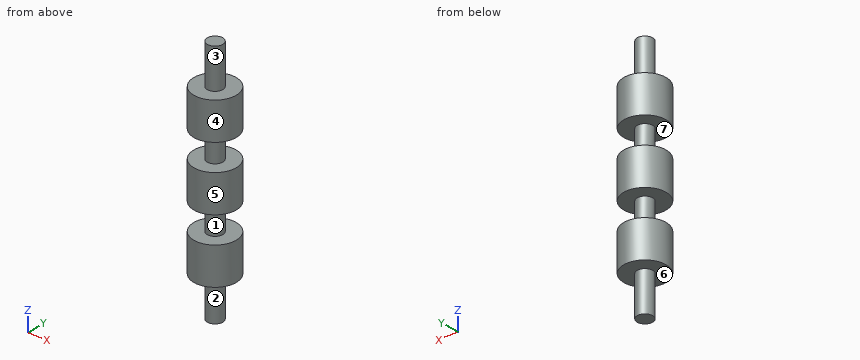
```python
from build123d import *

# Parameters (mm, degrees)
CROQUIS1_R              = 2.95
SALIENTE_EXTRUIR1_DEPTH = 15
CROQUIS2_R              = 8
SALIENTE_EXTRUIR2_DEPTH = 14
SALIENTE_EXTRUIR3_START = 10
CROQUIS3_R              = 2.95
SALIENTE_EXTRUIR3_DEPTH = 10
CROQUIS4_R              = 8
SALIENTE_EXTRUIR4_DEPTH = 14
SALIENTE_EXTRUIR5_START = 10
CROQUIS5_R              = 2.95
SALIENTE_EXTRUIR5_DEPTH = 10
CROQUIS6_R              = 8
SALIENTE_EXTRUIR6_DEPTH = 14
SALIENTE_EXTRUIR7_START = 15
CROQUIS7_R              = 2.95
SALIENTE_EXTRUIR7_DEPTH = 15


with BuildPart() as part:
    # Croquis1 → Saliente-Extruir1 (new body)
    with BuildSketch(Plane.XY):
        Circle(CROQUIS1_R)
    extrude(amount=SALIENTE_EXTRUIR1_DEPTH)

    # Croquis2 → Saliente-Extruir2 (add)
    with BuildSketch(Plane(origin=(0, 0, 0), x_dir=(-1, 0, 0), z_dir=(0, 0, -1))):
        Circle(CROQUIS2_R)
    extrude(amount=SALIENTE_EXTRUIR2_DEPTH)

    # Croquis3 → Saliente-Extruir3 (add)
    with BuildSketch(Plane(origin=(0, 0, -14), x_dir=(-1, 0, 0), z_dir=(0, 0, -1)).offset(SALIENTE_EXTRUIR3_START)):
        with Locations(Location((0, 0, 0), (0, 0, 180))):
            Circle(CROQUIS3_R)
    extrude(amount=-SALIENTE_EXTRUIR3_DEPTH)

    # Croquis4 → Saliente-Extruir4 (add)
    with BuildSketch(Plane(origin=(0, 0, -24), x_dir=(-1, 0, 0), z_dir=(0, 0, -1))):
        Circle(CROQUIS4_R)
    extrude(amount=SALIENTE_EXTRUIR4_DEPTH)

    # Croquis5 → Saliente-Extruir5 (add)
    with BuildSketch(Plane(origin=(0, 0, -38), x_dir=(-1, 0, 0), z_dir=(0, 0, -1)).offset(SALIENTE_EXTRUIR5_START)):
        with Locations(Location((0, 0, 0), (0, 0, 180))):
            Circle(CROQUIS5_R)
    extrude(amount=-SALIENTE_EXTRUIR5_DEPTH)

    # Croquis6 → Saliente-Extruir6 (add)
    with BuildSketch(Plane(origin=(0, 0, -48), x_dir=(-1, 0, 0), z_dir=(0, 0, -1))):
        Circle(CROQUIS6_R)
    extrude(amount=SALIENTE_EXTRUIR6_DEPTH)

    # Croquis7 → Saliente-Extruir7 (add)
    with BuildSketch(Plane(origin=(0, 0, -62), x_dir=(-1, 0, 0), z_dir=(0, 0, -1)).offset(SALIENTE_EXTRUIR7_START)):
        with Locations(Location((0, 0, 0), (0, 0, 180))):
            Circle(CROQUIS7_R)
    extrude(amount=-SALIENTE_EXTRUIR7_DEPTH)


solid = part.part
```
Input: part model. Units: mm. Frame: model coordinates. Face numbers are marked on the shaded views. A direction names the side the tool comes from. Give positions to 0.01 mm unless a question says otherwise; leave off trailing zeros. Loops run counter-clockwise (first coordinate to the right, second up) from the corner with the lowest first, then second, coordinate; pieces in that order, holes last. Notation, with made-up numbers: (89, -38.75) -> (134, -38.75) arc R21 cw to (134, -23.75) -> close; hole circle Ø9 at (-17.5, 19). An arc over 180 degrees is marked (long way). Use a Markdown table: item, result.
Q1. Ray query, probe 1 along Z at (x, y) = (5.5, 5); probe 2 along Y at (x, z) = (2.5, -32); probe 3 along Y at (x, z) = (1.75, -62.5). Return the intervals inside material, ascending. Write a range as from..to.
Entries:
| item | result |
|---|---|
| probe 1 | z = -62..-48, -38..-24, -14..0 |
| probe 2 | y = -7.6..7.6 |
| probe 3 | y = -2.37..2.37 |
Q2. Access query for the marked faces 1, 2, 3 and 4. Directions: +Z, -Z, +X, -X, +Y, -Y. A direction counts if a zero-diameter tool reaches every point of the face in a straight line with its end or side. Return the directions, or none.
Entries:
| item | result |
|---|---|
| face 1 | none |
| face 2 | -Z |
| face 3 | +Z |
| face 4 | +Z, -Z |
Q3. Section query B-B, the plane y = 6.25. Return the cut outline in (x, z).
Entries:
| item | result |
|---|---|
| outline | (-4.99, -62) -> (4.99, -62) -> (4.99, -48) -> (-4.99, -48) -> close; (-4.99, -38) -> (4.99, -38) -> (4.99, -24) -> (-4.99, -24) -> close; (-4.99, -14) -> (4.99, -14) -> (4.99, 0) -> (-4.99, 0) -> close |
Q4. First-contact query: P1, Ø5, axis at y = 2, z = -18.5, coming from the +X side; P2, Ø1, axis at x = -1.5, z = -2.5, coming from the -Y side; P3, Ø1.5, axis at x = 3, z = -52, coming from the +Y side. Flat tips, straight axial feed; report the tip coordinate or a pass-through.
Entries:
| item | result |
|---|---|
| P1 | stops at x = 2.95 |
| P2 | stops at y = -7.94 |
| P3 | stops at y = 7.68 |
Q5. Pull-direction query (Z, two-part tool) for the marked faces 5, 6 and 7; classes: pulls with the +Z half, pulls with the -Z half, needs draft (parallel to the pull), parting line crosses it, or undercut.
Entries:
| item | result |
|---|---|
| face 5 | needs draft |
| face 6 | pulls with the -Z half |
| face 7 | undercut |
Q6. Section query C-C, the plane x = 6. Return the cut outline in (y, z), plus the area to 3 significant figures.
Entries:
| item | result |
|---|---|
| outline | (-5.29, -62) -> (5.29, -62) -> (5.29, -48) -> (-5.29, -48) -> close; (-5.29, -38) -> (5.29, -38) -> (5.29, -24) -> (-5.29, -24) -> close; (-5.29, -14) -> (5.29, -14) -> (5.29, 0) -> (-5.29, 0) -> close |
| area | 444 mm² |
Q7. Section query A-A, the plane x = 0. Return the cut outline in (y, z), plus the area to 3 significant figures.
Entries:
| item | result |
|---|---|
| outline | (-8, -62) -> (-2.95, -62) -> (-2.95, -77) -> (2.95, -77) -> (2.95, -62) -> (8, -62) -> (8, -48) -> (2.95, -48) -> (2.95, -38) -> (8, -38) -> (8, -24) -> (2.95, -24) -> (2.95, -14) -> (8, -14) -> (8, 0) -> (2.95, 0) -> (2.95, 15) -> (-2.95, 15) -> (-2.95, 0) -> (-8, 0) -> (-8, -14) -> (-2.95, -14) -> (-2.95, -24) -> (-8, -24) -> (-8, -38) -> (-2.95, -38) -> (-2.95, -48) -> (-8, -48) -> close |
| area | 967 mm² |
